For this review, use the dimensioned drawing (mm, ordinates from the lowest corner) and the shaded views. A direction names the side the tool comes from. Round coordinates to 2 decimals unless told otherwise and drop trailing zeros. Write each loop counter-clockwise with the first axis right and the second up, starting at its lowest first coordinate (ties: lowest second). Pieces come first, ordered by that corner, then holes.
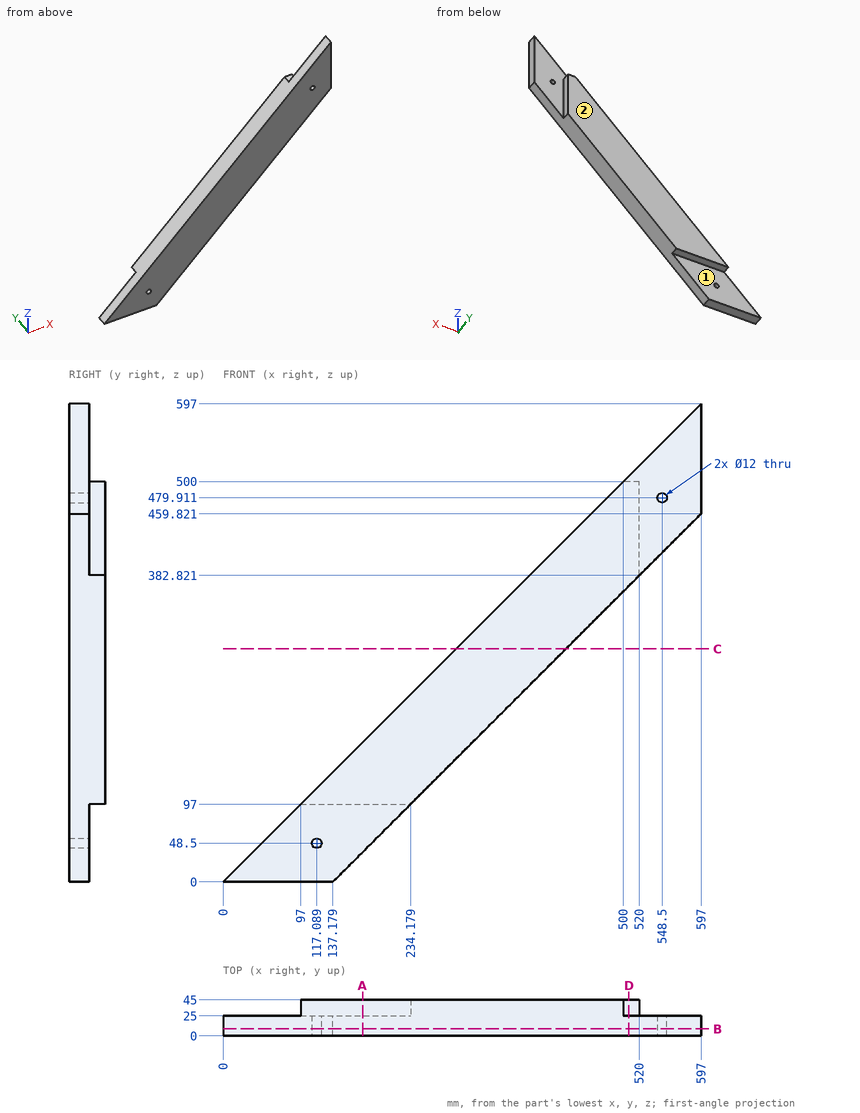
(1) We need section A-A, the plane x = 174.5. Give the boundary of the cut face in (y, z).
Geometry check:
outline: (0, 37.32) - (25, 37.32) - (25, 97) - (45, 97) - (45, 174.5) - (0, 174.5) - close
(2) For line 1 along Z through (x, y) = (260.5, 21.5); line 2 along Z through (x, y) = (92, 13.5); line 3 along X through (y, z) = (19.5, 164.5), list the stretches that pass through material, from the lowest coordinate up.
Geometry check:
line 1: z = 123.32 to 260.5
line 2: z = 0 to 92
line 3: x = 164.5 to 301.68
(3) We need section C-C, the plane z = 291. Give the boundary of the cut face in (x, y).
Geometry check:
outline: (291, 0) - (428.18, 0) - (428.18, 45) - (291, 45) - close
(4) For pin 1 Ø22 at (x, y) = (139.5, 40) entering from -Z; pin 2 Ø2 at (y, z) = (40, 333) entering from -X; pin 3 Ø3 at (x, y) = (400.5, 37) entering from +Z; pin 4 Ø7 at (x, z) = (548.5, 479.91) entering from +Y (1 decimal), all flat-tipped, find the tip position at first contact; note any pin that passes through.
Geometry check:
pin 1: stops at z = 97
pin 2: stops at x = 332
pin 3: stops at z = 402
pin 4: passes through
(5) We need section D-D, the plane x = 507. Give the boundary of the cut face in (y, z), and give its area (3 significant figures).
Geometry check:
outline: (0, 369.82) - (45, 369.82) - (45, 500) - (25, 500) - (25, 507) - (0, 507) - close
area: 6,030 mm2
(6) We need section B-B, the plane y = 9. Give the boundary of the cut face in (x, z), and give its area (3 significant figures).
Geometry check:
outline: (0, 0) - (137.18, 0) - (597, 459.82) - (597, 597) - close; hole circle Ø12 at (117.09, 48.5); hole circle Ø12 at (548.5, 479.91)
area: 72,300 mm2
(7) For the marked faces 1 and 2, list the 3-axis set-ups (+Z, -Z, +X, -X, +Y, -Y) from which the entire face can be reached by the end or side of a thin tool; tool diameter is ignored.
Geometry check:
face 1: -Z, +X, -X, +Y
face 2: +Z, -Z, +X, -X, +Y
